Can you work these out from the model? Positions are in its coordinate system, mm. Face numbers are marked on the shaded views. A direction names the side the tool comes from. Round coordinates to 2 decimals unless told otherwise and drop trailing zeros. Loops run counter-clockwise (first coordinate to the right, second up) from the corner with the lowest first, then second, coordinate; pieces in that order, holes last.
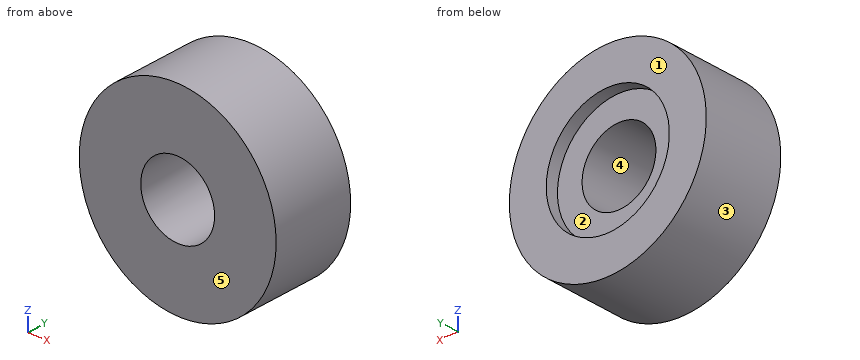
from build123d import *

# Parameters (mm, degrees)
ESQUISSE1_R             = 6
BOSS_EXTRU_1_DEPTH      = 5
ENL_V_MAT_EXTRU_1_REACH = 7
ESQUISSE2_R             = 2.25
ESQUISSE3_R             = 3.75
ENL_V_MAT_EXTRU_2_DEPTH = 0.75


with BuildPart() as part:
    # Esquisse1 → Boss.-Extru.1 (new body)
    with BuildSketch(Plane(origin=(0, 0, 0), x_dir=(1, 0, 0), z_dir=(0, 1, 0))):
        Circle(ESQUISSE1_R)
    extrude(amount=BOSS_EXTRU_1_DEPTH)

    # Esquisse2 → Enlèv. mat.-Extru.1 (cut, up to next)
    with BuildSketch(Plane(origin=(0, 5, 0), x_dir=(1, 0, 0), z_dir=(0, 1, 0)), mode=Mode.PRIVATE) as enl_v_mat_extru_1_sk1:
        Circle(ESQUISSE2_R)
    enl_v_mat_extru_1_tool1 = extrude(enl_v_mat_extru_1_sk1.sketch, amount=-ENL_V_MAT_EXTRU_1_REACH, mode=Mode.PRIVATE) & part.part
    add(enl_v_mat_extru_1_tool1.solids().sort_by_distance((0, 5, 0))[0], mode=Mode.SUBTRACT)

    # Esquisse3 → Enlèv. mat.-Extru.2 (cut)
    with BuildSketch(Plane(origin=(0, 5, 0), x_dir=(1, 0, 0), z_dir=(0, 1, 0))):
        Circle(ESQUISSE3_R)
    extrude(amount=-ENL_V_MAT_EXTRU_2_DEPTH, mode=Mode.SUBTRACT)


solid = part.part
(1) If we section it at A-A, the plane z = 0: List the corners of the cut face in (x, y) for me.
Worked answers:
outline: (-6, 0) - (-2.25, 0) - (-2.25, 4.25) - (-3.75, 4.25) - (-3.75, 5) - (-6, 5) - close; (2.25, 0) - (6, 0) - (6, 5) - (3.75, 5) - (3.75, 4.25) - (2.25, 4.25) - close
(2) If we mould it in two halves opening along X, with no side actions, what happens to the marked faces 3, 4 and 5? For each: released by +X, released by -X, zero draft, split by the parting line, or undercut.
Worked answers:
face 3: split by the parting line
face 4: undercut
face 5: zero draft
(3) If I drill on line 1 (X direction, y = 4.65, z = 0); line 2 (Z direction, x = 0, y = 2.3), over which ranges is the centre line in solid material (lowest first)?
Worked answers:
line 1: x = -6 to -3.75, 3.75 to 6
line 2: z = -6 to -2.25, 2.25 to 6
(4) If we section it at D-D, the plane y = 0.7: List the corners of the cut face in (x, z) for me, then the cut area to 3 significant figures.
Worked answers:
outline: circle Ø12 at (0, 0); hole circle Ø4.5 at (0, 0)
area: 97.2 mm2
(5) If we section it at B-B, the plane x = 0: List the corners of the cut face in (y, z) for me, then the cut area to 4 significant figures.
Worked answers:
outline: (0, -6) - (5, -6) - (5, -3.75) - (4.25, -3.75) - (4.25, -2.25) - (0, -2.25) - close; (0, 2.25) - (4.25, 2.25) - (4.25, 3.75) - (5, 3.75) - (5, 6) - (0, 6) - close
area: 35.25 mm2
(6) Will these pins go through, and if not, where does the flat tip stop? P1, Ø3, axis at x = 0.5, y = 4.5, coming from the -Z side; P2, Ø1, axis at x = 4, y = 2.5, coming from the -Z side.
Worked answers:
P1: stops at z = -6
P2: stops at z = -4.87
(7) For the marked faces 1 and 2, which set-ups out of +Z, -Z, +X, -X, +Y, -Y let a thin tool reach every point of the face, with its end or its side?
Worked answers:
face 1: +Z, -Z, +X, -X, +Y
face 2: +Y
(8) If we section it at C-C, the plane z = -2.5: List the corners of the cut face in (x, y) for me, then the cut area to 3 significant figures.
Worked answers:
outline: (-5.45, 0) - (5.45, 0) - (5.45, 5) - (2.8, 5) - (2.8, 4.25) - (-2.8, 4.25) - (-2.8, 5) - (-5.45, 5) - close
area: 50.4 mm2
